Could you check a few things on this model? Use its own coordinates, in mm. A direction names the side the tool comes from. Round coordinates to 2 decimals unless told otherwise and drop trailing zeros. Write each loop counter-clockwise with the first axis right and the second up, starting at its lowest first coordinate (ties: lowest second). Pieces come first, ordered by that corner, then holes. Notation, with made-up numbers: (-5, -19.5) -> (51, -19.5) arc R21 cw to (51, 14.5) -> close; hole circle Ø7 at (74, -14.75). An arc over 180 degrees is marked (long way). Answer as CSV lines item,"result". Start each with the question number.
Q1. If we mould it in two halves opening along Y, with no side actions, what happens to faces 5 (the flat face through (3, 0, 2)), 6 (the flat face through (3, 3, 0)), 7 (the flat face through (2.177, 3, 9)), 8 (the flat face through (3, 5.8, 2))? For each: pulls with the +Y half, pulls with the -Y half, needs draft (parallel to the pull), parting line crosses it, or undercut.
Q2. Imagine slicing it at A-A on x = 1.35. Please give me the cut outline in (y, z), and give its area (3 significant figures).
Q3. Imagine slicing it at D-D on z = 5.5. Please give me the cut outline in (x, y), and give its area (3 significant figures).
Q4. Imagine slicing it at B-B on y = 3.05. Please give me the cut outline in (x, z), and give its area (3 significant figures).
Q5. If I drill on line 1 (X direction, y = 0.6, z = -2.5); line 2 (Z direction, x = 1.95, y = 2.9); line 3 (Z direction, x = 4.45, y = 3.3), over which ranges is the centre line in solid material (lowest first)? Write a range as [from, to].
Q6. Imagine slicing it at C-C on y = 1.55. Please give me the cut outline in (x, z).
Q7. Will these pins go through, and if not, where does the flat tip stop? pin 1 Ø1.5 at (y, z) = (2.5, 7.5) entering from +X; pin 2 Ø0.6 at (x, z) = (3, 8) entering from +Y; pin 3 Ø0.5 at (y, z) = (2.5, 8) entering from -X.
Q8. For faces 1 (the flat face through (1.877, 3, 8)), 2 (the flat face through (3, 3.806, 9)), 3 (the flat face through (3, 1.994, 9)), 4 (the flat face through (3.923, 3, 8)), which set-ups out of +Z, -Z, +X, -X, +Y, -Y let a thin tool reach every point of the face, with its end or its side?
from build123d import *

# Parameters (mm, degrees)
SKETCH1_W           = 5.8
SKETCH1_H           = 5.8
BOSS_EXTRUDE2_DEPTH = 5
SKETCH3_W           = 3.5
SKETCH3_H           = 3
BOSS_EXTRUDE3_DEPTH = 2.5
SKETCH4_W           = 2.046388996
SKETCH4_H           = 1.811822668
BOSS_EXTRUDE4_DEPTH = 2.5
SKETCH5_W           = 0.5
SKETCH5_H           = 0.2
BOSS_EXTRUDE5_DEPTH = 3.6
SKETCH6_W           = 1
SKETCH6_H           = 0.3
SKETCH6_W_2         = 0.3
SKETCH6_H_2         = 1
CUT_EXTRUDE1_DEPTH  = 2


with BuildPart() as part:
    # Sketch1 → Boss-Extrude2 (new body)
    with BuildSketch(Plane.XY):
        with Locations((2.9, 2.9)):
            Rectangle(SKETCH1_W, SKETCH1_H)
    extrude(amount=BOSS_EXTRUDE2_DEPTH)

    # Sketch3 → Boss-Extrude3 (add)
    with BuildSketch(Plane.XY.offset(5)):
        with Locations((2.9, 2.9)):
            Rectangle(SKETCH3_W, SKETCH3_H)
    extrude(amount=BOSS_EXTRUDE3_DEPTH)

    # Sketch4 → Boss-Extrude4 (add)
    with BuildSketch(Plane.XY.offset(7.5)):
        with Locations((2.9, 2.9)):
            Rectangle(SKETCH4_W, SKETCH4_H)
    extrude(amount=BOSS_EXTRUDE4_DEPTH)

    # Sketch5 → Boss-Extrude5 (add)
    with BuildSketch(Plane(origin=(0, 0, 0), x_dir=(-1, 0, 0), z_dir=(0, 0, -1))):
        with Locations((-4.9, 5.15)):
            Rectangle(SKETCH5_W, SKETCH5_H)
        with Locations((-2.9, 5.15)):
            Rectangle(SKETCH5_W, SKETCH5_H)
        with Locations((-0.9, 5.15)):
            Rectangle(SKETCH5_W, SKETCH5_H)
        with Locations((-0.9, 0.65)):
            Rectangle(SKETCH5_W, SKETCH5_H)
        with Locations((-2.9, 0.65)):
            Rectangle(SKETCH5_W, SKETCH5_H)
        with Locations((-4.9, 0.65)):
            Rectangle(SKETCH5_W, SKETCH5_H)
    extrude(amount=BOSS_EXTRUDE5_DEPTH)

    # Sketch6 → Cut-Extrude1 (cut)
    with BuildSketch(Plane.XZ.offset(-1.994088666)):
        with Locations((2.901805502, 9.85)):
            Rectangle(SKETCH6_W, SKETCH6_H)
        with Locations((2.026805502, 8.9)):
            Rectangle(SKETCH6_W_2, SKETCH6_H_2)
        with Locations((3.773194498, 8.9)):
            Rectangle(SKETCH6_W_2, SKETCH6_H_2)
    extrude(amount=-CUT_EXTRUDE1_DEPTH, mode=Mode.SUBTRACT)


solid = part.part
Checks:
1,face 5,"pulls with the -Y half"
1,face 6,"undercut"
1,face 7,"needs draft"
1,face 8,"pulls with the +Y half"
2,outline,"(0, 0) -> (5.8, 0) -> (5.8, 5) -> (4.4, 5) -> (4.4, 7.5) -> (1.4, 7.5) -> (1.4, 5) -> (0, 5) -> close"
2,area,"36.5 mm^2"
3,outline,"(1.15, 1.4) -> (4.65, 1.4) -> (4.65, 4.4) -> (1.15, 4.4) -> close"
3,area,"10.5 mm^2"
4,outline,"(0, 0) -> (5.8, 0) -> (5.8, 5) -> (4.65, 5) -> (4.65, 7.5) -> (3.92, 7.5) -> (3.92, 8.4) -> (3.62, 8.4) -> (3.62, 9.4) -> (3.92, 9.4) -> (3.92, 10) -> (3.4, 10) -> (3.4, 9.7) -> (2.4, 9.7) -> (2.4, 10) -> (1.88, 10) -> (1.88, 9.4) -> (2.18, 9.4) -> (2.18, 8.4) -> (1.88, 8.4) -> (1.88, 7.5) -> (1.15, 7.5) -> (1.15, 5) -> (0, 5) -> close"
4,area,"42.0 mm^2"
5,line 1,"[0.65, 1.15], [2.65, 3.15], [4.65, 5.15]"
5,line 2,"[0, 8.4], [9.4, 10]"
5,line 3,"[0, 7.5]"
6,outline,"(0, 0) -> (5.8, 0) -> (5.8, 5) -> (4.65, 5) -> (4.65, 7.5) -> (1.15, 7.5) -> (1.15, 5) -> (0, 5) -> close"
7,pin 1,"x = 4.65"
7,pin 2,"y = 3.81"
7,pin 3,"x = 1.88"
8,face 1,"+Z, -X, +Y, -Y"
8,face 2,"+Z, +X, -X, +Y"
8,face 3,"+Z, +X, -X, -Y"
8,face 4,"+Z, +X, +Y, -Y"
